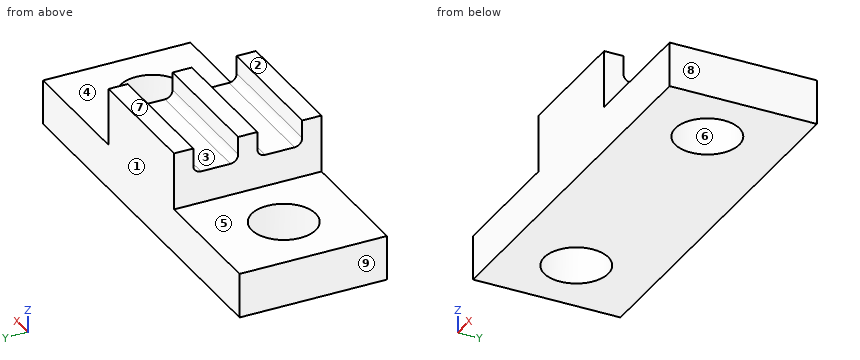
```python
from build123d import *

# Parameters (mm, degrees)
SKETCH1_W              = 30
SKETCH1_H              = 11.5
SKETCH1_R              = 2.5
BOSS_EXTRUDE1_DEPTH    = 3.5
SKETCH2_W              = 10
SKETCH2_H              = 11.5
BOSS_EXTRUDE2_DEPTH    = 4.5
SKETCH3_W              = 2
SKETCH3_H              = 3.5
CUT_EXTRUDE1_DEPTH     = 23.29489852
FILLET1_R              = 0.6
LPATTERN1_COUNT        = 2
LPATTERN1_PITCH        = 5
FILLET1_OF_LPATTERN1_R = 0.6


with BuildPart() as part:
    # Sketch1 → Boss-Extrude1 (new body)
    with BuildSketch(Plane.XY):
        Rectangle(SKETCH1_W, SKETCH1_H)
        with Locations((-10, -0.25)):
            Circle(SKETCH1_R, mode=Mode.SUBTRACT)
        with Locations((10, -0.25)):
            Circle(SKETCH1_R, mode=Mode.SUBTRACT)
    extrude(amount=BOSS_EXTRUDE1_DEPTH)

    # Sketch2 → Boss-Extrude2 (add)
    with BuildSketch(Plane.XY.offset(3.5)):
        Rectangle(SKETCH2_W, SKETCH2_H)
    extrude(amount=BOSS_EXTRUDE2_DEPTH)

    # Sketch3 → Cut-Extrude1 (cut, through all)
    with BuildSketch(Plane.ZY.offset(5)):
        with Locations((7, 2.5)):
            Rectangle(SKETCH3_W, SKETCH3_H)
    cut_extrude1 = extrude(amount=-CUT_EXTRUDE1_DEPTH, mode=Mode.SUBTRACT)

    # Fillet1
    fillet1_edges = [part.edges().sort_by_distance(p)[0] for p in [
        (0, 0.75, 6),
        (0, 4.25, 6),
    ]]
    fillet(fillet1_edges, radius=FILLET1_R)

    # LPattern1: Cut-Extrude1 ×2
    with Locations(*[(0, -i * LPATTERN1_PITCH, 0) for i in range(1, LPATTERN1_COUNT)]):
        add(cut_extrude1, mode=Mode.SUBTRACT)

    # Fillet1 of LPattern1
    fillet1_of_lpattern1_edges = [part.edges().sort_by_distance(p)[0] for p in [
        (0, -4.25, 6),
        (0, -0.75, 6),
    ]]
    fillet(fillet1_of_lpattern1_edges, radius=FILLET1_OF_LPATTERN1_R)


solid = part.part
```
The model under review builds one solid part; all positions refer to its coordinate system, in mm. Face numbers are marked on the shaded views. A direction names the side the tool comes from. Round coordinates to 2 decimals unless told otherwise and drop trailing zeros. Loops run counter-clockwise (first coordinate to the right, second up) from the corner with the lowest first, then second, coordinate; pieces in that order, holes last. Notation, with made-up numbers: (33.5, 26.5) - (92.5, 26.5) arc R24 ccw to (92.5, 62.5) - close; hole circle Ø7 at (52, -36.75). An arc over 180 degrees is marked (long way). Use a Markdown table: item, result. Add a question column.
Q1. Insertion check: pin 1 Ø1.3 at (y, z) = (2, 5) entering from +X; pin 2 Ø1.2 at (x, y) = (1, 3) entering from +Z; pin 3 Ø1.3 at (y, z) = (-2, 5.5) entering from -X. Each pin has a flat end and moves straight along its axis. Give the tip position at first contact, or say it passes through.
Q2. Add section C-C (y = -2.25). State the section outline as (x, z) points.
Q3. Machinability: for the marked faces 1, 2, 3, 4 and 5, which of the approach directions +Z, -Z, +X, -X, +Y, -Y give a long, thin tool a straight path to every point of the face, cutting with its end or side? Answer none if there is none.
Q4. Add section B-B (y = -0.25). State the section outline as (x, z) points.
Q5. For probe 1 along Y at (x, z) = (-10, 1.05); probe 2 along Y at (x, z) = (2, 6.75); probe 3 along Z at (x, y) = (-13, 3.25), list the stretches that pass through material, from the lowest coordinate up.
Q6. Add section A-A (x = -10). State the section outline as (y, z) points.
Q7. The part is to be moulded in two halves that separate along X. For the marked faces 6, 7, 8 and 9, say which applies: pulls with the +X half, pulls with the -X half, needs draft (parallel to the pull), parting line crosses it, or undercut.
Q8. Add section D-D (x = -0.25). State the section outline as (y, z) points, plus the area to 3 significant figures.
Worked answers:
| question | item | result |
|---|---|---|
| 1 | pin 1 | x = 5 |
| 1 | pin 2 | z = 6 |
| 1 | pin 3 | x = -5 |
| 2 | outline | (-15, 0) - (-11.5, 0) - (-11.5, 3.5) - (-15, 3.5) - close; (-8.5, 0) - (8.5, 0) - (8.5, 3.5) - (5, 3.5) - (5, 6) - (-5, 6) - (-5, 3.5) - (-8.5, 3.5) - close; (11.5, 0) - (15, 0) - (15, 3.5) - (11.5, 3.5) - close |
| 3 | face 1 | +Z, -Z, +X, -X, +Y |
| 3 | face 2 | +Z, +X, -X, +Y, -Y |
| 3 | face 3 | +Z, +X, -X |
| 3 | face 4 | +Z, +X, +Y, -Y |
| 3 | face 5 | +Z, -X, +Y, -Y |
| 4 | outline | (-15, 0) - (-12.5, 0) - (-12.5, 3.5) - (-15, 3.5) - close; (-7.5, 0) - (7.5, 0) - (7.5, 3.5) - (5, 3.5) - (5, 8) - (-5, 8) - (-5, 3.5) - (-7.5, 3.5) - close; (12.5, 0) - (15, 0) - (15, 3.5) - (12.5, 3.5) - close |
| 5 | probe 1 | -5.75 to -2.75, 2.25 to 5.75 |
| 5 | probe 2 | -5.75 to -4.25, -0.75 to 0.75, 4.25 to 5.75 |
| 5 | probe 3 | 0 to 3.5 |
| 6 | outline | (-5.75, 0) - (-2.75, 0) - (-2.75, 3.5) - (-5.75, 3.5) - close; (2.25, 0) - (5.75, 0) - (5.75, 3.5) - (2.25, 3.5) - close |
| 7 | face 6 | undercut |
| 7 | face 7 | needs draft |
| 7 | face 8 | pulls with the +X half |
| 7 | face 9 | pulls with the -X half |
| 8 | outline | (-5.75, 0) - (5.75, 0) - (5.75, 8) - (4.25, 8) - (4.25, 6.6) arc R0.6 cw to (3.65, 6) - (1.35, 6) arc R0.6 cw to (0.75, 6.6) - (0.75, 8) - (-0.75, 8) - (-0.75, 6.6) arc R0.6 cw to (-1.35, 6) - (-3.65, 6) arc R0.6 cw to (-4.25, 6.6) - (-4.25, 8) - (-5.75, 8) - close |
| 8 | area | 78.3 mm² |
